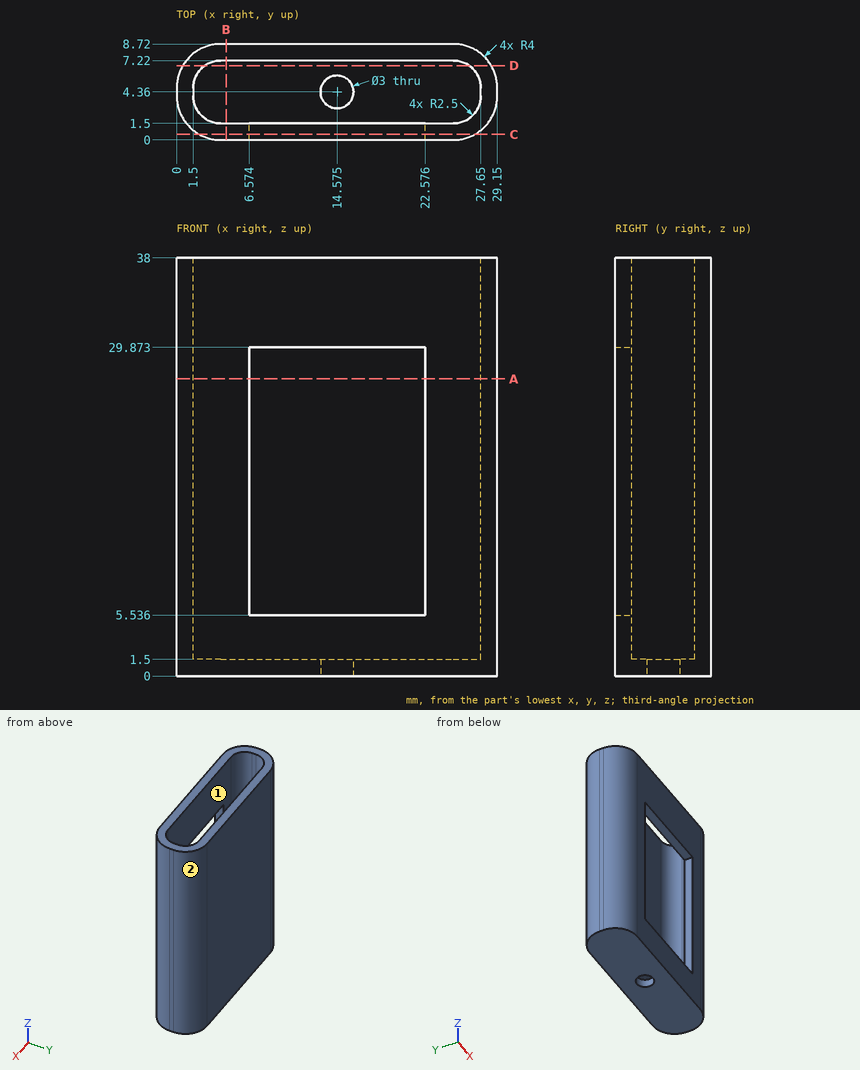
Answer from the drawing. Dimensions are ordinates in mm from the lowest x, y and z of the part. A direction names the side the tool comes from. Give positions to 0.01 mm unless a question says otherwise; leave off trailing zeros. Write each loop counter-clockwise with the first axis right and the second up, starting at its lowest first coordinate (ties: lowest second). Pieces come first, ordered by that corner, then holes. Notation, with made-up numbers: (73.25, 84) -> (126.25, 84) arc R15 ccw to (126.25, 107) -> close; hole circle Ø6 at (46.25, -16.5). An arc over 180 degrees is marked (long way). One line per question, with ' | ' between items. Start each with the question number.
1. Section D-D (y = 6.75) is taken. Determine the outline of the cut face in (x, z), plus the area to 3 significant figures.
2. Section B-B (x = 4.5) is taken. Determine the outline of the cut face in (y, z).
3. Given pin 1 Ø1.7 at (x, y) = (13, 5) entering from +Z; pin 2 Ø1.6 at (y, z) = (0.5, 13.5) entering from +X; pin 3 Ø1.6 at (y, z) = (0.5, 14.5) entering from -X, each flat-ended and moving along its own axis, determine where each tip first touches the part or whether it passes through.
4. Find the intervals of material crossed by probe 1 along X at (y, z) = (4.5, 20); probe 2 along Y at (x, z) = (14.25, 32), in increasing order.
5. Section A-A (z = 27) is taken. Determine the outline of the cut face in (x, y).
6. Section C-C (y = 0.5) is taken. Determine the outline of the cut face in (x, z) (1 decimal).
7. For the marked faces 1 and 2, determine the directions among +Z, -Z, +X, -X, +Y, -Y from which every point of the face is accessible in a straight line to the end or side of a thin tool.
Response values:
1) outline: (0.55, 0) -> (28.6, 0) -> (28.6, 38) -> (26.61, 38) -> (26.61, 1.5) -> (2.54, 1.5) -> (2.54, 38) -> (0.55, 38) -> close | area: 187 mm2
2) outline: (0, 0) -> (8.72, 0) -> (8.72, 38) -> (7.22, 38) -> (7.22, 1.5) -> (1.5, 1.5) -> (1.5, 38) -> (0, 38) -> close
3) pin 1: z = 1.5 | pin 2: x = 28.1 | pin 3: x = 1.05
4) probe 1: 0 to 1.5, 27.65 to 29.15 | probe 2: 0 to 1.5, 7.22 to 8.72
5) outline: (0, 4) arc R4 ccw to (4, 0) -> (6.57, 0) -> (6.57, 1.5) -> (4, 1.5) arc R2.5 cw to (1.5, 4) -> (1.5, 4.72) arc R2.5 cw to (4, 7.22) -> (25.15, 7.22) arc R2.5 cw to (27.65, 4.72) -> (27.65, 4) arc R2.5 cw to (25.15, 1.5) -> (22.58, 1.5) -> (22.58, 0) -> (25.15, 0) arc R4 ccw to (29.15, 4) -> (29.15, 4.72) arc R4 ccw to (25.15, 8.72) -> (4, 8.72) arc R4 ccw to (0, 4.72) -> close
6) outline: (2.1, 0) -> (27.1, 0) -> (27.1, 38) -> (2.1, 38) -> close; hole (6.6, 5.5) -> (22.6, 5.5) -> (22.6, 29.9) -> (6.6, 29.9) -> close
7) face 1: +Z | face 2: +Z, -Z, +X, +Y
